The listing builds one solid part. Answer for the finished solid, in the listing's coordinates (mm). A direction names the side the tool comes from. Give positions to 0.01 mm unless a question says otherwise; leave off trailing zeros. Write each loop counter-clockwise with the first axis right and the second up, starting at its lowest first coordinate (ties: lowest second). Pieces come first, ordered by that corner, then holes. Notation, with made-up numbers: M 58.25,-23.5 L 93.25,-23.5 A22 cw 93.25,10.5 Z; hole C 19,9.5 d9. An arc over 180 degrees is marked long. Answer as a JSON object with one key per item and string values.
```python
from build123d import *

# Parameters (mm, degrees)
SKETCH_1_W               = 250
SKETCH_1_H               = 60
EXTRUDE_1_DEPTH          = 10
FILLET_1_R               = 20
SKETCH_5_R               = 10
CUT_EXTRUDE_3_DEPTH      = 10
SKETCH_15_R              = 14.25
CUT_EXTRUDE_12_DEPTH     = 129.937969582
SKETCH_18_R              = 1.3
CUT_EXTRUDE_14_DEPTH     = 129.937969582
CUT_EXTRUDE_15_DEPTH     = 129.937969582
SKETCH_20_R              = 2
CUT_EXTRUDE_16_DEPTH     = 10
SKETCH_21_R              = 2.1
CUT_EXTRUDE_17_DEPTH     = 10
CUT_EXTRUDE_18_DEPTH     = 129.937969582
PATTERN_CIRCULAR_1_COUNT = 4


with BuildPart() as part:
    # 草图1 → 凸台-拉伸1 (new body)
    with BuildSketch(Plane(origin=(0, 0, 0), x_dir=(1, 0, 0), z_dir=(0, 1, 0))):
        Rectangle(SKETCH_1_W, SKETCH_1_H)
    extrude(amount=EXTRUDE_1_DEPTH)

    # 圆角1
    fillet_1_edges = [part.edges().sort_by_distance(p)[0] for p in [
        (125, 5, 30),
        (-125, 5, 30),
        (-125, 5, -30),
        (125, 5, -30),
    ]]
    fillet(fillet_1_edges, radius=FILLET_1_R)

    # 草图5 → 切除-拉伸3 (cut)
    with BuildSketch(Plane.XZ):
        with Locations(Location((-100, 0, 0), (0, 0, 270))):
            Circle(SKETCH_5_R)
    extrude(amount=-CUT_EXTRUDE_3_DEPTH, mode=Mode.SUBTRACT)

    # 草图15 → 切除-拉伸12 (cut, through all)
    with BuildSketch(Plane.XZ):
        with Locations(Location((95, 0, 0), (0, 0, 270))):
            Circle(SKETCH_15_R)
    extrude(amount=-CUT_EXTRUDE_12_DEPTH, mode=Mode.SUBTRACT)

    # 草图18 → 切除-拉伸14 (cut, through all)
    with BuildSketch(Plane.XZ):
        with Locations(Location((82.625631329, 12.374368671, 0), (0, 0, 270))):
            Circle(SKETCH_18_R)
        with Locations(Location((107.374368671, 12.374368671, 0), (0, 0, 270))):
            Circle(SKETCH_18_R)
        with Locations(Location((107.374368671, -12.374368671, 0), (0, 0, 270))):
            Circle(SKETCH_18_R)
        with Locations(Location((82.625631329, -12.374368671, 0), (0, 0, 270))):
            Circle(SKETCH_18_R)
    extrude(amount=-CUT_EXTRUDE_14_DEPTH, mode=Mode.SUBTRACT)

    # 草图19 → 切除-拉伸15 (cut, through all)
    with BuildSketch(Plane(origin=(0, 0, 0), x_dir=(-1, 0, 0), z_dir=(0, -1, 0))):
        with BuildLine():
            Line((62.26537952, 17), (52.26537952, 17))
            ThreePointArc((52.26537952, 17), (50.76537952, 15.5), (52.26537952, 14))
            Line((52.26537952, 14), (62.26537952, 14))
            ThreePointArc((62.26537952, 14), (63.76537952, 15.5), (62.26537952, 17))
        make_face()
        with BuildLine():
            Line((31.26537952, -17), (21.26537952, -17))
            ThreePointArc((21.26537952, -17), (19.76537952, -15.5), (21.26537952, -14))
            Line((21.26537952, -14), (31.26537952, -14))
            ThreePointArc((31.26537952, -14), (32.76537952, -15.5), (31.26537952, -17))
        make_face()
        with BuildLine():
            Line((31.26537952, 17), (21.26537952, 17))
            ThreePointArc((21.26537952, 17), (19.76537952, 15.5), (21.26537952, 14))
            Line((21.26537952, 14), (31.26537952, 14))
            ThreePointArc((31.26537952, 14), (32.76537952, 15.5), (31.26537952, 17))
        make_face()
        with BuildLine():
            Line((62.26537952, -17), (52.26537952, -17))
            ThreePointArc((52.26537952, -17), (50.76537952, -15.5), (52.26537952, -14))
            Line((52.26537952, -14), (62.26537952, -14))
            ThreePointArc((62.26537952, -14), (63.76537952, -15.5), (62.26537952, -17))
        make_face()
    extrude(amount=-CUT_EXTRUDE_15_DEPTH, mode=Mode.SUBTRACT)

    # 草图20 → 切除-拉伸16 (cut)
    with BuildSketch(Plane(origin=(0, 10, 0), x_dir=(1, 0, 0), z_dir=(0, 1, 0))):
        with Locations(Location((-100, 17.5, 0), (0, 0, 270))):
            Circle(SKETCH_20_R)
    cut_extrude_16 = extrude(amount=-CUT_EXTRUDE_16_DEPTH, mode=Mode.SUBTRACT)

    # 草图21 → 切除-拉伸17 (cut)
    with BuildSketch(Plane.XZ):
        with Locations(Location((95, 17.5, 0), (0, 0, 270))):
            Circle(SKETCH_21_R)
        with Locations(Location((112.5, 0, 0), (0, 0, 270))):
            Circle(SKETCH_21_R)
        with Locations(Location((95, -17.5, 0), (0, 0, 270))):
            Circle(SKETCH_21_R)
        with Locations(Location((77.5, 0, 0), (0, 0, 270))):
            Circle(SKETCH_21_R)
    extrude(amount=-CUT_EXTRUDE_17_DEPTH, mode=Mode.SUBTRACT)

    # 草图22 → 切除-拉伸18 (cut, through all)
    with BuildSketch(Plane(origin=(0, 10, 0), x_dir=(1, 0, 0), z_dir=(0, 1, 0))):
        with BuildLine():
            Line((0, 15), (50, 15))
            ThreePointArc((50, 15), (65, 0), (50, -15))
            Line((50, -15), (0, -15))
            ThreePointArc((0, -15), (-15, 0), (0, 15))
        make_face()
    extrude(amount=-CUT_EXTRUDE_18_DEPTH, mode=Mode.SUBTRACT)

    # 阵列(圆周)1: 切除-拉伸16 ×4 about axis
    pattern_circular_1_axis = Axis((-100, 0, 0), (0, 1, 0))
    for i in range(1, PATTERN_CIRCULAR_1_COUNT):
        add(cut_extrude_16.rotate(pattern_circular_1_axis, i * 360 / PATTERN_CIRCULAR_1_COUNT), mode=Mode.SUBTRACT)


solid = part.part
```
1. A cutting plane is placed at D-D, the plane y = 7. Count the separate pieces of the cut face and the enclosed holes in it, plus the area to 3 significant figures.
Verdict:
{"separate pieces": "1", "enclosed holes": "19", "area": "11,200 mm2"}
2. The mould has two halves that part along Z. Classify faces 3 (the flat face through (-1, 5, 30)), 4 (the flat face through (-57, 5, 14)), 5 (the flat face through (-30, 0, 0)): released by +Z, released by -Z, zero draft, split by the parting line, or undercut.
Verdict:
{"face 3": "released by +Z", "face 4": "undercut", "face 5": "zero draft"}
3. A cutting plane is placed at B-B, the plane x = 95. Give the vertices of the cut face in (y, z).
Verdict:
{"outline": "M 0,-30 L 10,-30 L 10,-19.6 L 0,-19.6 Z; M 0,-15.4 L 10,-15.4 L 10,-14.25 L 0,-14.25 Z; M 0,14.25 L 10,14.25 L 10,15.4 L 0,15.4 Z; M 0,19.6 L 10,19.6 L 10,30 L 0,30 Z"}
4. A cutting plane is placed at A-A, the plane x = -107.5. Give the vertices of the cut face in (y, z).
Verdict:
{"outline": "M 0,-29.84 L 10,-29.84 L 10,-6.61 L 0,-6.61 Z; M 0,6.61 L 10,6.61 L 10,29.84 L 0,29.84 Z"}
5. Flat-ended cylindrical pins translate along their axes: pin 1 (4.5 mm diameter, centred on x = -82.5, z = 0, fed in from +Y); pin 2 (5 mm diameter, centred on y = 1, z = 14.5, fed in from -X). Find the tip coordinate at first contact, or state that the pin passes through.
Verdict:
{"pin 1": "stops at y = 10", "pin 2": "stops at x = -124.9"}
6. For faces 1 (the flat face through (-30, 10, 0)), 2 (the flat face through (25, 5, -15)), determine the directions among +Z, -Z, +X, -X, +Y, -Y from which every point of the face is accessible in a straight line to the end or side of a thin tool.
Verdict:
{"face 1": "+Z, -Z, +X, -X, +Y", "face 2": "+Y, -Y"}
7. A cutting plane is placed at C-C, the plane z = 23. Give the vertices of the cut face in (x, y).
Verdict:
{"outline": "M -120.2,0 L 120.2,0 L 120.2,10 L -120.2,10 Z"}
8. Consider line 1 along Z through (x, y) = (-28, 6.5); line 2 along Z through (x, y) = (28.5, 5.75); line 3 along X through (y, z) = (3, -4). Determine where each line is inside the solid, lowest interval first.
Verdict:
{"line 1": "z = -30 to -17, -14 to 14, 17 to 30", "line 2": "z = -30 to -15, 15 to 30", "line 3": "x = -125 to -109.17, -90.83 to -14.46, 64.46 to 81.32, 108.68 to 125"}
